from build123d import *

# Parameters (mm, degrees)
SKETCH1_W               = 50
SKETCH1_H               = 50
BOSS_EXTRUDE1_DEPTH     = 15
SHELL2_T                = -2
CUT_EXTRUDE1_DEPTH      = 39.405728739
CUT_EXTRUDE1_DEPTH_BACK = 39.405728739
SKETCH3_R               = 10
FILLET1_R               = 2
FILLET3_R               = 2
SKETCH5_R               = 2.5
SKETCH5_R_2             = 1.5
BOSS_EXTRUDE2_DEPTH     = 3
LPATTERN2_COUNT         = 2
LPATTERN2_PITCH         = 20
LPATTERN2_COUNT_DIR2    = 2
LPATTERN2_PITCH_DIR2    = 35


with BuildPart() as part:
    # Sketch1 → Boss-Extrude1 (new body)
    with BuildSketch(Plane(origin=(0, 0, 0), x_dir=(0, 1, 0), z_dir=(0, 0, 1))):
        Rectangle(SKETCH1_W, SKETCH1_H)
    extrude(amount=BOSS_EXTRUDE1_DEPTH)

    # Shell2
    shell2_openings = [part.faces().sort_by_distance(p)[0] for p in [
        (0, 0, 0),
    ]]
    offset(amount=SHELL2_T, openings=shell2_openings, kind=Kind.INTERSECTION)

    # Sketch3 → Cut-Extrude1 (cut, two sides: drawn at the far end of the back side and taken through both)
    with BuildSketch(Plane.XY.offset(15).offset(-CUT_EXTRUDE1_DEPTH_BACK)):
        with Locations(Location((0, 0, 0), (0, 0, 180))):
            Circle(SKETCH3_R)
    extrude(amount=CUT_EXTRUDE1_DEPTH + CUT_EXTRUDE1_DEPTH_BACK, mode=Mode.SUBTRACT)

    # Fillet1
    fillet1_edges = [part.edges().sort_by_distance(p)[0] for p in [
        (23, 23, 6.5),
        (-23, 23, 6.5),
        (-23, -23, 6.5),
        (23, -23, 6.5),
    ]]
    fillet(fillet1_edges, radius=FILLET1_R)

    # Fillet3
    fillet3_edges = [part.edges().sort_by_distance(p)[0] for p in [
        (25, 25, 7.5),
        (25, -25, 7.5),
        (-25, -25, 7.5),
        (-25, 25, 7.5),
    ]]
    fillet(fillet3_edges, radius=FILLET3_R)

    # Sketch5 → Boss-Extrude2 (add)
    with BuildSketch(Plane(origin=(0, 0, 13), x_dir=(1, 0, 0), z_dir=(0, 0, -1))):
        with Locations(Location((17.5, 10, 0), (0, 0, 180))):
            Circle(SKETCH5_R)
        with Locations(Location((17.5, 10, 0), (0, 0, 180))):
            Circle(SKETCH5_R_2, mode=Mode.SUBTRACT)
    boss_extrude2 = extrude(amount=BOSS_EXTRUDE2_DEPTH)

    # LPattern2: Boss-Extrude2 2 × 2
    with Locations(*[(-j * LPATTERN2_PITCH_DIR2, i * LPATTERN2_PITCH, 0) for i in range(LPATTERN2_COUNT) for j in range(LPATTERN2_COUNT_DIR2) if (i, j) != (0, 0)]):
        add(boss_extrude2)


solid = part.part
Here's how the part is built. I have some questions about the finished solid (model axes, mm). A direction names the side the tool comes from. Give positions to 0.01 mm unless a question says otherwise; leave off trailing zeros. Write each loop counter-clockwise with the first axis right and the second up, starting at its lowest first coordinate (ties: lowest second). Pieces come first, ordered by that corner, then holes. Notation, with made-up numbers: (52.25, 58) -> (91.25, 58) arc R22 ccw to (91.25, 89) -> close; hole circle Ø9 at (-19.5, -20). An arc over 180 degrees is marked (long way). Use one line per item in the form item = value. Start each with the question number.
1. Imagine slicing it at A-A on z = 6.75. List the corners of the cut face in (x, y) for me.
2. Will these pins go through, and if not, where does the flat tip stop? pin 1 Ø1.5 at (x, y) = (17.5, 9) entering from -Z; pin 2 Ø0.9 at (x, y) = (17.5, -10.5) entering from -Z.
3. If I drill on L1, parallel to Y at x = -17.5, z = 10.75; L2, parallel to Y at x = 13, z = 1.5; L3, parallel to Y at x = 0, z = 14.35, over which ranges is the centre line in solid material (lowest first)?
4. Thinking about a two-plate mould opening in Y: for faces 1 (the face through (24.43, 24.4, 7.6)), 2 (the face through (-24.4, -24.43, 7.6)), 3 (the face through (10, 0, 14)), which applies, +Y half, -Y half, draft (parallel to the pull), parting line (faces both ways), or undercut?
5. On a 3-axis mill with a long thin cutter (end or side, diameter ignored), from which of +Z, -Z, +X, -X, +Y, -Y can I reach the whole of each face in a straight line? I mean faces 4 (the face through (-25, 0, 7)), 5 (the face through (19, -10, 12)). Say none if no direction works.
6. Imagine slicing it at B-B on x = 0. List the corners of the cut face in (y, z) for me, plus the area to 3 significant figures.
7. Imagine slicing it at C-C on y = 19. List the corners of the cut face in (x, z) for me, plus the area to 3 significant figures.
Entries:
q1.outline = (-25, -23) arc R2 ccw to (-23, -25) -> (23, -25) arc R2 ccw to (25, -23) -> (25, 23) arc R2 ccw to (23, 25) -> (-23, 25) arc R2 ccw to (-25, 23) -> close; hole (-23, -21) arc R2 ccw to (-21, -23) -> (21, -23) arc R2 ccw to (23, -21) -> (23, 21) arc R2 ccw to (21, 23) -> (-21, 23) arc R2 ccw to (-23, 21) -> close
q2.pin_1 = 10
q2.pin_2 = 13
q3.L1 = -25 to -23, -12.5 to -11.5, -8.5 to -7.5, 7.5 to 8.5, 11.5 to 12.5, 23 to 25
q3.L2 = -25 to -23, 23 to 25
q3.L3 = -25 to -10, 10 to 25
q4.face_1 = +Y half
q4.face_2 = -Y half
q4.face_3 = undercut
q5.face_4 = +Z, -Z, -X, +Y, -Y
q5.face_5 = -Z
q6.outline = (-25, 0) -> (-23, 0) -> (-23, 13) -> (-10, 13) -> (-10, 15) -> (-25, 15) -> close; (10, 13) -> (23, 13) -> (23, 0) -> (25, 0) -> (25, 15) -> (10, 15) -> close
q6.area = 112 mm²
q7.outline = (-25, 0) -> (-23, 0) -> (-23, 13) -> (23, 13) -> (23, 0) -> (25, 0) -> (25, 15) -> (-25, 15) -> close
q7.area = 152 mm²
